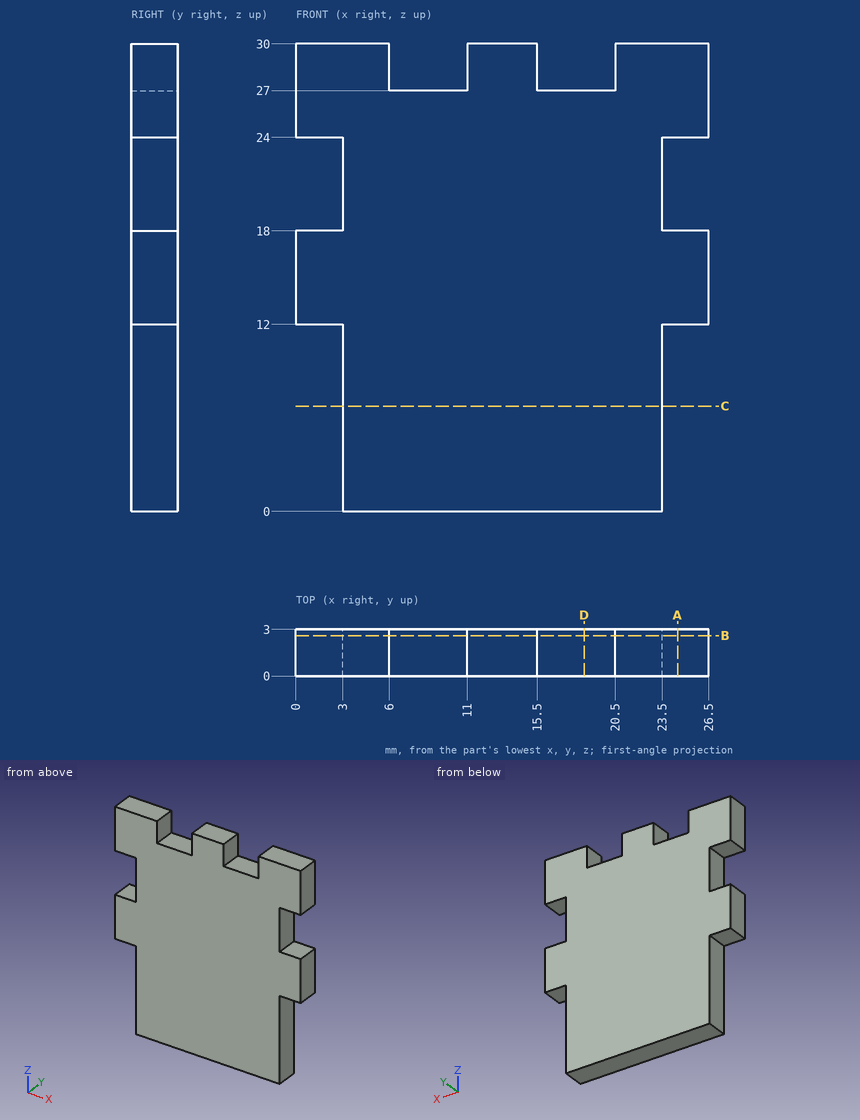
Study the drawing (mm; zero at the part's minimum x, y, z) and answer. Give positions to 0.01 mm unless a question says otherwise; leave off trailing zeros. Order: outer loops, then holes, each group sorted by start corner. A loop starts at its lowest first (then second) coordinate and runs counter-clockwise, first axis right, second up. Notation, with made-up numbers: (52, 81.5) - (59, 81.5) arc R33 ccw to (59, 119.5) - close; hole circle Ø2 at (25, 23). An arc over 180 degrees is marked (long way). Use one line per item in the form item = value. Start each with the question number.
(1) Flat-ended cylindrical pins translate along their axes: pin 1 Ø1.5 at (x, y) = (24.5, 1) entering from -Z; pin 2 Ø0.9 at (y, z) = (1.5, 21.5) entering from +X; pin 3 Ø0.9 at (x, y) = (18, 2) entering from +Z. Find the tip coordinate at first contact, or state that the pin passes through.
(2) A cutting plane is placed at A-A, the plane x = 24.5. Write down the section's boundary in (y, z).
(3) A cutting plane is placed at B-B, the plane y = 2.6. Write down the section's boundary in (x, z).
(4) A cutting plane is placed at C-C, the plane z = 6.75. Write down the section's boundary in (x, y), then the cut area to 3 significant figures.
(5) A cutting plane is placed at D-D, the plane x = 18.5. Write down the section's boundary in (y, z).
(6) Consider line 1 (X direction, y = 1.35, z = 28); line 2 (Z direction, x = 23.75, y = 0.85); line 3 (X direction, y = 2.45, z = 23.5). Determine where each line is inside the solid, lowest interval first. Write a range as from..to.
Ans:
q1.pin_1 = 12
q1.pin_2 = 23.5
q1.pin_3 = 27
q2.outline = (0, 12) - (3, 12) - (3, 18) - (0, 18) - close; (0, 24) - (3, 24) - (3, 30) - (0, 30) - close
q3.outline = (0, 12) - (3, 12) - (3, 0) - (23.5, 0) - (23.5, 12) - (26.5, 12) - (26.5, 18) - (23.5, 18) - (23.5, 24) - (26.5, 24) - (26.5, 30) - (20.5, 30) - (20.5, 27) - (15.5, 27) - (15.5, 30) - (11, 30) - (11, 27) - (6, 27) - (6, 30) - (0, 30) - (0, 24) - (3, 24) - (3, 18) - (0, 18) - close
q4.outline = (3, 0) - (23.5, 0) - (23.5, 3) - (3, 3) - close
q4.area = 61.5 mm^2
q5.outline = (0, 0) - (3, 0) - (3, 27) - (0, 27) - close
q6.line_1 = 0..6, 11..15.5, 20.5..26.5
q6.line_2 = 12..18, 24..30
q6.line_3 = 3..23.5
